Autodesk Inventor part; units mm, degrees
ref_plane "YZ Plane" through (0, 0, 0) normal (1, 0, 0) x (0, 1, 0)
ref_plane "XZ Plane" through (0, 0, 0) normal (0, 1, 0) x (-1, 0, 0)
ref_plane "XY Plane" through (0, 0, 0) normal (0, 0, 1) x (1, 0, 0)
sketch "スケッチ1" plane through (0, 0, 0) normal (0, 0, 1) x (1, 0, 0)
  circle A0 centre (0, 0) radius 4
  dimension "d0" = 8
extrude "押し出し1" add sketch "スケッチ1" along normal blind 1
sketch "スケッチ2" plane through (0, 0, 1) normal (0, 0, 1) x (1, 0, 0)
  circle A0 centre (0, 0) radius 2.5
  dimension "d3" = 5
extrude "押し出し2" add sketch "スケッチ2" along normal blind 5
sketch "スケッチ3" plane through (0, 0, 6) normal (0, 0, 1) x (1, 0, 0)
  point P0 (0, 0)
  point P1 (0, 0)
hole "穴1" at (0, 0, 6) direction (0, 0, -1) diameter 3 end through all
sketch "スケッチ4" plane through (0, 0, 6) normal (0, 0, 1) x (1, 0, 0)
  circle A0 centre (0, 0) radius 2.5
extrude "押し出し3" cut sketch "スケッチ4" against normal up to surface (5 mm away)
properties part number "RD017"
Geometry check sheet. Reference: the model listing, model coordinates, mm. Give positions to 0.01 mm unless a question says otherwise; leave off trailing zeros. Loops run counter-clockwise (first coordinate to the right, second up) from the corner with the lowest first, then second, coordinate; pieces in that order, holes last. Notation, with made-up numbers: M -32.5,7 L -7.5,7 A29 ccw -7.5,29 Z; hole C 66.25,39 d11. An arc over 180 degrees is marked long. Write each question's results on one line, items separated by ' | '.
1) Section check A-A, the plane y = 0. Record the boundary of the cut face in (x, z), plus the area to 3 significant figures.
Answers follow:
outline: M -4,0 L -1.5,0 L -1.5,1 L -4,1 Z; M 1.5,0 L 4,0 L 4,1 L 1.5,1 Z | area: 5.00 mm2
2) Thickness scan on line 1 (Y direction, x = 0, z = 0.65); line 2 (Y direction, x = 0.5, z = 0.35); line 3 (X direction, y = 3.25, z = 0.95). Record the ranges inside material, lowest first.
Answers follow:
line 1: -4 to -1.5, 1.5 to 4 | line 2: -3.97 to -1.41, 1.41 to 3.97 | line 3: -2.33 to 2.33
3) Section check D-D, the plane y = 2.5. Record the boundary of the cut face in (x, z), plus the area to 4 significant figures.
Answers follow:
outline: M -3.12,0 L 3.12,0 L 3.12,1 L -3.12,1 Z | area: 6.245 mm2
4) Section check C-C, the plane z = 0.45. Record the boundary of the cut face in (x, y).
Answers follow:
outline: C 0,0 d8; hole C 0,0 d3
